Work out the finished part from the listing and answer in its coordinate system (mm). Round coordinates to 2 decimals unless told otherwise and drop trailing zeros. Order: outer loops, then holes, each group sorted by start corner. A loop starts at its lowest first (then second) coordinate and runs counter-clockwise, first axis right, second up. Notation, with made-up numbers: (-6.5, 40.25) - (39.5, 40.25) arc R23 cw to (39.5, 50.25) - close; hole circle Ø6 at (78, 21.5). An arc over 180 degrees is marked (long way). Use one line per item in the form item = value. Start each with the question number.
Q1. The part is cut by section A-A on y = 12. Determine the outline of the cut face in (x, z).
Q2. The part is cut by section B-B on y = -19. Determine the outline of the cut face in (x, z), plus the area to 3 significant figures.
Q3. Find the intervals of material crossed by line 1 (X direction, y = 13, z = 5.75); line 2 (X direction, y = 17.5, z = 1); line 3 (Z direction, x = -4.5, y = -8), in increasing order. Write a range as [from, to].
Q4. Given P1, Ø8, axis at x = 5.5, y = 8, coming from the -Z side; P2, Ø3, axis at y = 6, z = -3.5, coming from the +X side; P3, Ø4, axis at y = -21.5, z = -1, coming from the +X side, each flat-ended and moving along its own axis, determine where each tip first touches the part or whether it passes through.
from build123d import *

# Parameters (mm, degrees)
SKETCH_606_R    = 8
EXTRUDE_1_DEPTH = 24


# Read off the part's stored shape, not the designer's step: 凸台-拉伸2
with BuildPart() as part:
    # Sketch 606 → 凸台-拉伸1 (new body)
    with BuildSketch(Plane(origin=(0, 0, 0), x_dir=(1, 0, 0), z_dir=(0, 1, 0))):
        with Locations(Location((0, 0, 0), (0, 0, 270))):
            Circle(SKETCH_606_R)
    extrude(amount=EXTRUDE_1_DEPTH)

    # 凸台-拉伸2 outline → 凸台-拉伸2 (revolve)
    with BuildSketch(Plane.XY):
        Polygon((0, -23), (6.794621076, -23), (8, 0), (0, 0), align=None)
    revolve(axis=Axis((0, 0, 0), (0, 1, 0)))

    # 草图7 → 旋转4 (revolve)
    with BuildSketch(Plane.XY, mode=Mode.PRIVATE) as revolve_4_sk:
        with BuildLine():
            Line((0, -23), (6.794621076, -23))
            Line((6.794621076, -23), (4.608094813, -40.807827362))
            ThreePointArc((4.608094813, -40.807827362), (3.408750419, -43.087406102), (1, -44))
            Line((1, -44), (0, -44))
            Line((0, -44), (0, -23))
        make_face()
    revolve(revolve_4_sk.sketch.rotate(Axis((0, -23, 0), (0, -1, 0)), 180), axis=Axis((0, -23, 0), (0, -1, 0)))


solid = part.part
Found:
q1.outline = circle Ø16 at (0, 0)
q2.outline = circle Ø14.01 at (0, 0)
q2.area = 154 mm²
q3.line_1 = [-5.56, 5.56]
q3.line_2 = [-7.94, 7.94]
q3.line_3 = [-6.1, 6.1]
q4.P1 = -7.86
q4.P2 = 7.75
q4.P3 = 6.97
